Part model, mm, in its own coordinate system. Face numbers are marked on the shaded views. Coordinates: 2 decimals unless noted, no trailing zeros. Loops run counter-clockwise (first coordinate to the right, second up) from the corner with the lowest first, then second, coordinate; pieces in that order, holes last. Notation, with made-up numbers: M 52,85 L 99,85 A27 cw 99,117 Z; hole C 42.5,77 d9. An arc over 180 degrees is marked long. Use a Markdown table: item, result. Add a question column.
1) Band-saw the part on A-A (x = 9). List the corners of the cut face in (y, z).
2) Pull direction Z, two halves, no side cores. Call the marked faces 1 and 2: released by +Z, released by -Z, zero draft, split by the parting line, or undercut.
3) Pin check, flat tips, straight feed: pin 1 Ø4 at (y, z) = (2, -2) entering from -X; pin 2 Ø2 at (x, z) = (-7.5, -1.5) entering from +Y; pin 3 Ø1.5 at (x, y) = (-5, -4.5) entering from +Z. Stop position of each tip, or through.
4) Wall check: probe 1 along Z at (x, y) = (-4.25, 0); probe 2 along X at (y, z) = (-5, 3); probe 3 along Z at (x, y) = (5.75, 1.75). Give the ranges that are in metal, low to high. Write a range as from..to.
Autodesk Inventor part; units mm, degrees
ref_plane "YZ Plane" through (0, 0, 0) normal (1, 0, 0) x (0, 1, 0)
ref_plane "XZ Plane" through (0, 0, 0) normal (0, 1, 0) x (-1, 0, 0)
ref_plane "XY Plane" through (0, 0, 0) normal (0, 0, 1) x (1, 0, 0)
sketch "Эскиз1" plane through (0, 0, 0) normal (1, 0, 0) x (0, 1, 0)
  circle A0 centre (0, 0) radius 7.5
  circle A1 centre (0, 0) radius 4
  dimension "d0" = 15
  dimension "d1" = 8
extrude "Выдавливание1" add sketch "Эскиз1" along normal mid plane 24
sketch "Эскиз2" plane through (12, 0, 0) normal (1, 0, 0) x (0, 0, -1)
  circle A0 centre (0, 0) radius 5
  circle A1 centre (0, 0) radius 6.5
  dimension "d4" = 10
  dimension "d5" = 13
extrude "Выдавливание2" cut sketch "Эскиз2" against normal blind 1
sketch "Эскиз3" plane through (-12, 0, 0) normal (-1, 0, 0) x (0, 0, 1)
  circle A0 centre (0, 0) radius 6.5
  circle A1 centre (0, 0) radius 5
  dimension "d9" = 13
  dimension "d10" = 10
extrude "Выдавливание3" cut sketch "Эскиз3" against normal blind 1
fillet "Сопряжение1" radius 0.5 1 edges at (-12, -7.5, 0)
fillet "Сопряжение2" radius 0.5 3 edges at (-12, -4, 0) (12, -7.5, 0) (12, -4, 0)
chamfer "Фаска1" distance 0.2 angle 45 8 edges at (12, 0, 5) (12, 0, 6.5) (-12, 0, -5) (-12, 0, -6.5) (-11, 0, -5) (-11, 0, -6.5) (11, 0, 6.5) (11, 0, 5)
properties part number "LM8UU"
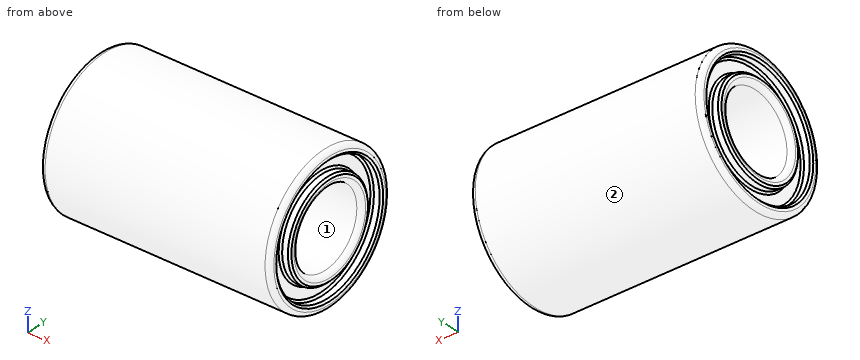
Entries:
| question | item | result |
|---|---|---|
| 1 | outline | C 0,0 d15; hole C 0,0 d8 |
| 2 | face 1 | undercut |
| 2 | face 2 | split by the parting line |
| 3 | pin 1 | x = -12 |
| 3 | pin 2 | y = 7.48 |
| 3 | pin 3 | z = 6.5 |
| 4 | probe 1 | -7.5..-4, 4..7.5 |
| 4 | probe 2 | -11..11 |
| 4 | probe 3 | -7.29..-3.6, 3.6..7.29 |
